```python
from build123d import *

# Parameters (mm, degrees)
SKETCH1_W           = 40
SKETCH1_H           = 18
BOSS_EXTRUDE1_DEPTH = 7.5
SKETCH2_R           = 1.7
CUT_EXTRUDE1_DEPTH  = 24.178653973
SKETCH3_R           = 1.7
CUT_EXTRUDE2_DEPTH  = 25.5


with BuildPart() as part:
    # Sketch1 → Boss-Extrude1 (new body)
    with BuildSketch(Plane.XY):
        Rectangle(SKETCH1_W, SKETCH1_H)
    extrude(amount=BOSS_EXTRUDE1_DEPTH)

    # Sketch2 → Cut-Extrude1 (cut, through all)
    with BuildSketch(Plane(origin=(0, 0, 0), x_dir=(-1, 0, 0), z_dir=(0, 0, -1))):
        with Locations((-16, 4)):
            Circle(SKETCH2_R)
        with Locations((-16, -4)):
            Circle(SKETCH2_R)
        with Locations((16, 4)):
            Circle(SKETCH2_R)
        with Locations((16, -4)):
            Circle(SKETCH2_R)
        Polygon((10, -3), (14, -9), (-14, -9), (-10, -3), align=None)
        Polygon((-14, 9), (-10, 3), (10, 3), (14, 9), align=None)
    extrude(amount=-CUT_EXTRUDE1_DEPTH, mode=Mode.SUBTRACT)

    # Sketch3 → Cut-Extrude2 (cut, through all)
    with BuildSketch(Plane(origin=(0, 3, 0), x_dir=(1, 0, 0), z_dir=(0, 1, 0))):
        with Locations(Location((-5, -3.5, 0), (0, 0, 270))):
            Circle(SKETCH3_R)
        with Locations(Location((5, -3.5, 0), (0, 0, 270))):
            Circle(SKETCH3_R)
    extrude(amount=-CUT_EXTRUDE2_DEPTH, mode=Mode.SUBTRACT)


solid = part.part
```
Input: part model. Units: mm. Frame: model coordinates. A direction names the side the tool comes from. Round coordinates to 2 decimals unless told otherwise and drop trailing zeros. Order: outer loops, then holes, each group sorted by start corner. A loop starts at its lowest first (then second) coordinate and runs counter-clockwise, first axis right, second up. Notation, with made-up numbers: (32.25, -4) - (87.25, -4) arc R22 cw to (87.25, 10) - close; hole circle Ø1 at (-6, 7). An arc over 180 degrees is marked (long way). Answer in a Markdown table with one row per item.
Item 1: Line query: line 1 (X direction, y = 0.2, z = 3.5); line 2 (Y direction, x = 16, z = 3.5); line 3 (X direction, y = 4.25, z = 7). Output: solid intervals per line, ascending.
Model answer:
| item | result |
|---|---|
| line 1 | x = -20 to -6.7, -3.3 to 3.3, 6.7 to 20 |
| line 2 | y = -9 to -5.7, -2.3 to 2.3, 5.7 to 9 |
| line 3 | x = -20 to -17.68, -14.32 to -10.83, 10.83 to 14.32, 17.68 to 20 |
Item 2: Section query B-B (y = -7.5). Return the cut outline in (x, z).
Model answer:
| item | result |
|---|---|
| outline | (-20, 0) - (-13, 0) - (-13, 7.5) - (-20, 7.5) - close; (13, 0) - (20, 0) - (20, 7.5) - (13, 7.5) - close |
Item 3: Pin query (flat end, axial travel): pin 1 (4 mm diameter, centred on x = -4.5, z = 2, fed in from +Y); pin 2 (2 mm diameter, centred on x = 16, y = 4, fed in from -Z); pin 3 (4 mm diameter, centred on x = -3, z = 3.5, fed in from -Y). Return the tip coordinate at first contact, or that it passes through.
Model answer:
| item | result |
|---|---|
| pin 1 | stops at y = 3 |
| pin 2 | passes through |
| pin 3 | stops at y = -3 |
Item 4: Reachability of faces 4 (the flat face through (-12, -6, 4)), 5 (the flat face through (-12, 6, 4)), 6 (the flat face through (0, 0, 0)) from +Z, -Z, +X, -X, +Y, -Y: full face, straight path, thin tool, end or side. Return the list, or none.
Model answer:
| item | result |
|---|---|
| face 4 | +Z, -Z, -Y |
| face 5 | +Z, -Z, +Y |
| face 6 | -Z, +X, -X, +Y, -Y |
Item 5: Section query D-D (y = -4). Return the cut outline in (x, z), then the cut area to 3 significant figures.
Model answer:
| item | result |
|---|---|
| outline | (-20, 0) - (-17.7, 0) - (-17.7, 7.5) - (-20, 7.5) - close; (-14.3, 0) - (-10.67, 0) - (-10.67, 7.5) - (-14.3, 7.5) - close; (10.67, 0) - (14.3, 0) - (14.3, 7.5) - (10.67, 7.5) - close; (17.7, 0) - (20, 0) - (20, 7.5) - (17.7, 7.5) - close |
| area | 89.0 mm² |
Item 6: Section query A-A (z = 3.5). Return the cut outline in (x, y), then the cut area to 3 significant figures.
Model answer:
| item | result |
|---|---|
| outline | (-20, -9) - (-14, -9) - (-10, -3) - (-6.7, -3) - (-6.7, 3) - (-10, 3) - (-14, 9) - (-20, 9) - close; (-3.3, -3) - (3.3, -3) - (3.3, 3) - (-3.3, 3) - close; (6.7, -3) - (10, -3) - (14, -9) - (20, -9) - (20, 9) - (14, 9) - (10, 3) - (6.7, 3) - close; hole circle Ø3.4 at (-16, -4); hole circle Ø3.4 at (-16, 4); hole circle Ø3.4 at (16, -4); hole circle Ø3.4 at (16, 4) |
| area | 355 mm² |
Item 7: Mould query, pull axis X, two halves, no side actions, for faces 1 (the cylindrical face through (-17.57, 3.35, 3.7)), 2 (the flat face through (-17, -9, 4)), 3 (the flat face through (20, 0, 4)). Classes: released by +X, released by -X, zero draft, split by the parting line, or undercut.
Model answer:
| item | result |
|---|---|
| face 1 | undercut |
| face 2 | zero draft |
| face 3 | released by +X |
Item 8: Section query C-C (x = -16). Return the cut outline in (y, z).
Model answer:
| item | result |
|---|---|
| outline | (-9, 0) - (-5.7, 0) - (-5.7, 7.5) - (-9, 7.5) - close; (-2.3, 0) - (2.3, 0) - (2.3, 7.5) - (-2.3, 7.5) - close; (5.7, 0) - (9, 0) - (9, 7.5) - (5.7, 7.5) - close |
